Here's how the part is built. I have some questions about the finished solid (model axes, mm). A direction names the side the tool comes from. Give positions to 0.01 mm unless a question says otherwise; leave off trailing zeros. Loops run counter-clockwise (first coordinate to the right, second up) from the corner with the lowest first, then second, coordinate; pieces in that order, holes last. Notation, with made-up numbers: (-20.75, 33.5) - (37.25, 33.5) arc R17 cw to (37.25, 51.5) - close; hole circle Ø6 at (17.5, 37.5). An arc over 180 degrees is marked (long way). Use a Markdown table: item, result.
from build123d import *
from build123d.topology import SkipClean

# Parameters (mm, degrees)
SKETCH1_R           = 27.5
SKETCH1_R_2         = 17.5
BOSS_EXTRUDE1_DEPTH = 8
BOSS_EXTRUDE2_DEPTH = 7
SKETCH4_R           = 5
CUT_EXTRUDE1_DEPTH  = 40.705163392


with BuildPart() as part:
    # Sketch1 → Boss-Extrude1 (new body)
    with BuildSketch(Plane.XY):
        Circle(SKETCH1_R)
        Circle(SKETCH1_R_2, mode=Mode.SUBTRACT)
    extrude(amount=BOSS_EXTRUDE1_DEPTH)

    # Sketch2 → Boss-Extrude2 (add)
    with SkipClean():  # the faces are left unmerged after this step: merging them gives an invalid solid
        with BuildSketch(Plane.XY.offset(8)):
            with BuildLine():
                ThreePointArc((10.453586197, 14.034690435), (16.644995589, 15.807064972), (16.187563711, 22.230896993))
                ThreePointArc((16.187563711, 22.230896993), (10.533073102, 25.40284179), (4.293124723, 27.162825334))
                ThreePointArc((4.293124723, 27.162825334), (-0.575744113, 22.947498772), (2.54487111, 17.313972133))
                ThreePointArc((2.54487111, 17.313972133), (6.702864701, 16.165444776), (10.453586197, 14.034690435))
            make_face()
            with BuildLine():
                ThreePointArc((-17.38119155, 2.03572599), (-22.011817619, 6.51145654), (-27.3463034, 2.903392903))
                ThreePointArc((-27.3463034, 2.903392903), (-27.26604287, -3.579512009), (-25.670259139, -9.863457595))
                ThreePointArc((-25.670259139, -9.863457595), (-19.585244834, -11.972358414), (-16.266775263, -6.453063036))
                ThreePointArc((-16.266775263, -6.453063036), (-17.35111819, -2.277871278), (-17.38119155, 2.03572599))
            make_face()
            with BuildLine():
                ThreePointArc((21.377134416, -17.299367738), (20.160988946, -10.975140359), (13.721904153, -10.860909097))
                ThreePointArc((13.721904153, -10.860909097), (10.648253489, -13.887573497), (6.927605353, -16.070416425))
                ThreePointArc((6.927605353, -16.070416425), (5.36682203, -22.318521512), (11.158739689, -25.134289896))
                ThreePointArc((11.158739689, -25.134289896), (16.732969768, -21.823329781), (21.377134416, -17.299367738))
            make_face()
        extrude(amount=BOSS_EXTRUDE2_DEPTH)

    # Sketch4 → Cut-Extrude1 (cut, through all)
    with SkipClean():  # the faces are left unmerged after this step: merging them gives an invalid solid
        with BuildSketch(Plane.XY.offset(8)):
            with Locations((27.26604287, 3.579512009)):
                Circle(SKETCH4_R)
        extrude(amount=-CUT_EXTRUDE1_DEPTH, mode=Mode.SUBTRACT)


solid = part.part
(1) We'd pull the mould along Y, two halves only. Please class faces 1 (the face through (-13, 13, 0)), 2 (the face through (16.59, 15.73, 11.45)), 3 (the face through (-21.9, 6.5, 11.5)): pulls with the +Y half, pulls with the -Y half, needs draft (parallel to the pull), parting line crosses it, or undercut.
A:
| item | result |
|---|---|
| face 1 | needs draft |
| face 2 | undercut |
| face 3 | pulls with the +Y half |
(2) Suppose I cut it at B-B on y = 11. Write out the boundary of the cut face in (x, z), plus the area to 3 significant figures.
A:
| item | result |
|---|---|
| outline | (-25.2, 0) - (-13.61, 0) - (-13.61, 8) - (-25.2, 8) - close; (13.61, 0) - (25.2, 0) - (25.2, 8) - (13.61, 8) - close |
| area | 185 mm2 |
(3) Suppose I cut it at A-A on z = 10. Write out the boundary of the cut face in (x, y).
A:
| item | result |
|---|---|
| outline | (-27.35, 2.9) arc R27.5 ccw to (-25.67, -9.86) arc R5.11 ccw to (-16.27, -6.45) arc R17.5 cw to (-17.38, 2.04) arc R5.11 ccw to start; (2.54, 17.31) arc R17.5 cw to (10.45, 14.03) arc R5.11 ccw to (16.19, 22.23) arc R27.5 ccw to (4.29, 27.16) arc R5.11 ccw to start; (6.93, -16.07) arc R5.11 ccw to (11.16, -25.13) arc R27.5 ccw to (21.38, -17.3) arc R5.11 ccw to (13.72, -10.86) arc R17.5 cw to start |
(4) Suppose I cut it at D-D on y = -21.5. Write out the boundary of the cut face in (x, z).
A:
| item | result |
|---|---|
| outline | (-17.15, 0) - (17.15, 0) - (17.15, 15) - (5.07, 15) - (5.07, 8) - (-17.15, 8) - close |
(5) On a 3-axis mill with a long thin cutter (end or side, diameter ignored), from which of +Z, -Z, +X, -X, +Y, -Y can I reach the whole of each face in a straight line? I mean faces 4 (the face through (-0.56, 23.04, 11.45)), 5 (the face through (-22, -3, 15)), 6 (the face through (20.235, -11.039, 11.451)). Say none if no direction works.
A:
| item | result |
|---|---|
| face 4 | +Z, -X |
| face 5 | +Z, +X, -X, +Y, -Y |
| face 6 | +Z |
(6) If I drill on line 1 (Y direction, x = 0, z = 1.5); line 2 (Z direction, x = 19, y = 4.5); line 3 (X direction, y = 0, z = 4), over which ranges is the centre line in solid material (lowest first)?
A:
| item | result |
|---|---|
| line 1 | -27.5 to -17.5, 17.5 to 27.5 |
| line 2 | 0 to 8 |
| line 3 | -27.5 to -17.5, 17.5 to 23.78 |
(7) Suppose I cut it at C-C on x = -10. Write out the boundary of the cut face in (y, z), plus the area to 3 significant figures.
A:
| item | result |
|---|---|
| outline | (-25.62, 0) - (-14.36, 0) - (-14.36, 8) - (-25.62, 8) - close; (14.36, 0) - (25.62, 0) - (25.62, 8) - (14.36, 8) - close |
| area | 180 mm2 |
(8) Will these pins go through, and if not, where does the flat tip stop? pin 1 (12 mm diameter, centred on x = 15.5, y = 2, fed in from +Z); pin 2 (5 mm diameter, centred on y = -17, z = 8, fed in from -X).
A:
| item | result |
|---|---|
| pin 1 | z = 8 |
| pin 2 | x = -23.37 |
